Autodesk Inventor part; units mm, degrees
ref_plane "YZ Plane" through (0, 0, 0) normal (1, 0, 0) x (0, 1, 0)
ref_plane "XZ Plane" through (0, 0, 0) normal (0, 1, 0) x (-1, 0, 0)
ref_plane "XY Plane" through (0, 0, 0) normal (0, 0, 1) x (1, 0, 0)
sketch "Skizze_1" plane through (0, 0, 0) normal (0, 0, 1) x (1, 0, 0)
  arc A0 (-7.7, 0.5) -> (-7.5, 0.3) centre (-7.5, 0.5) ccw
  line L0 (-7.5, 0.3) -> (5.5, 0.3)
  arc A1 (5.5, 0.3) -> (5.7, 0.5) centre (5.5, 0.5) ccw
  line L1 (5.7, 0.5) -> (5.7, 10.1162)
  arc A2 (5.7, 10.1162) -> (5.581, 10.44) centre (5.2, 10.1162) ccw
  line L2 (5.581, 10.44) -> (4.1497, 12.1238)
  arc A3 (4.1497, 12.1238) -> (3.7688, 12.3) centre (3.7688, 11.8) ccw
  line L3 (3.7688, 12.3) -> (-7.2, 12.3)
  arc A4 (-7.2, 12.3) -> (-7.7, 11.8) centre (-7.2, 11.8) ccw
  line L4 (-7.7, 11.8) -> (-7.7, 0.5)
extrude "Extrusion1" add sketch "Skizze_1" along normal blind 7
sketch "Skizze_2" plane through (0, 0, 7) normal (0, 0, 1) x (1, 0, 0)
  line L0 (4.2, 0) -> (5.5, 0)
  arc A0 (5.5, 0) -> (5.7, 0.2) centre (5.5, 0.2) ccw
  line L1 (5.7, 0.2) -> (5.7, 0.5)
  line L2 (5.7, 0.5) -> (4.2, 0.5)
  line L3 (4.2, 0.5) -> (4.2, 0)
extrude "Extrusion2" add sketch "Skizze_2" against normal blind 0.8
pattern_linear "Rectangular Pattern1" count 2 spacing 3.5 along (0, 0, -1) of "Extrusion2"
sketch "Skizze_4" plane through (0, 0, 7) normal (0, 0, 1) x (1, 0, 0)
  line L0 (-7.7, 1) -> (-7.7, 0.2)
  arc A0 (-7.7, 0.2) -> (-7.5, 0) centre (-7.5, 0.2) ccw
  line L1 (-7.5, 0) -> (-5.7, 0)
  line L2 (-5.7, 0) -> (-5.7, 1)
  line L3 (-5.7, 1) -> (-7.7, 1)
extrude "Extrusion3" add sketch "Skizze_4" against normal blind 0.8
pattern_linear "Rectangular Pattern2" count 2 spacing 3.5 along (0, 0, -1) of "Extrusion3"
sketch "Skizze_6" plane through (0, 0, 7) normal (0, 0, 1) x (1, 0, 0)
  line L0 (-3.4, 0) -> (2.3, 0)
  line L1 (2.3, 0) -> (2.3, 1)
  line L2 (2.3, 1) -> (-3.4, 1)
  line L3 (-3.4, 1) -> (-3.4, 0)
extrude "Extrusion4" add sketch "Skizze_6" against normal blind 0.8
pattern_linear "Rectangular Pattern3" count 2 spacing 3.5 along (0, 0, -1) of "Extrusion4"
sketch "Skizze_8" plane through (0, 0, 0) normal (0, 0, 1) x (1, 0, 0)
  circle A0 centre (4.3, 1.6) radius 0.6
extrude "Extrusion5" add sketch "Skizze_8" against normal blind 1.5
sketch "Skizze_9" plane through (0, 0, 0) normal (0, 0, 1) x (1, 0, 0)
  circle A0 centre (4.3, 4.7) radius 0.6
extrude "Extrusion6" add sketch "Skizze_9" against normal blind 1.5
sketch "Skizze_10" plane through (0, 0, 0) normal (0, 0, 1) x (1, 0, 0)
  circle A0 centre (4.3, 8.3) radius 0.6
extrude "Extrusion7" add sketch "Skizze_10" against normal blind 1.5
sketch "Skizze_11" plane through (0, 0, 0) normal (0, 0, 1) x (1, 0, 0)
  circle A0 centre (-6, 1.6) radius 0.5
extrude "Extrusion8" add sketch "Skizze_11" against normal blind 1.5
sketch "Skizze_12" plane through (0, 0, 0) normal (0, 0, 1) x (1, 0, 0)
  circle A0 centre (-6, 3.4) radius 0.5
extrude "Extrusion9" add sketch "Skizze_12" against normal blind 1.5
sketch "Skizze_13" plane through (0, 0, 0) normal (0, 0, 1) x (1, 0, 0)
  circle A0 centre (-6.5, 8.9) radius 0.5
extrude "Extrusion10" add sketch "Skizze_13" against normal blind 1.5
sketch "Skizze_14" plane through (0, 0, 0) normal (0, 0, 1) x (1, 0, 0)
  circle A0 centre (-6.5, 10.8) radius 0.5
extrude "Extrusion11" add sketch "Skizze_14" against normal blind 1.5
sketch "Skizze_15" plane through (0, 0, 0) normal (0, 0, 1) x (1, 0, 0)
  arc A0 (-7.7, 0.2) -> (-7.5, 0) centre (-7.5, 0.2) ccw
  line L0 (-7.5, 0) -> (-5.7, 0)
  line L1 (-5.7, 0) -> (-5.7, 0.3)
  line L2 (-5.7, 0.3) -> (-3.4, 0.3)
  line L3 (-3.4, 0.3) -> (-3.4, 0)
  line L4 (-3.4, 0) -> (2.3, 0)
  line L5 (2.3, 0) -> (2.3, 0.3)
  line L6 (2.3, 0.3) -> (4.2, 0.3)
  line L7 (4.2, 0.3) -> (4.2, 0)
  line L8 (4.2, 0) -> (5.5, 0)
  arc A1 (5.5, 0) -> (5.7, 0.2) centre (5.5, 0.2) ccw
  line L9 (5.7, 0.2) -> (5.7, 10.1162)
  arc A2 (5.7, 10.1162) -> (5.581, 10.44) centre (5.2, 10.1162) ccw
  line L10 (5.581, 10.44) -> (4.1497, 12.1238)
  arc A3 (4.1497, 12.1238) -> (3.7688, 12.3) centre (3.7688, 11.8) ccw
  line L11 (3.7688, 12.3) -> (-7.2, 12.3)
  arc A4 (-7.2, 12.3) -> (-7.7, 11.8) centre (-7.2, 11.8) ccw
  line L12 (-7.7, 11.8) -> (-7.7, 0.2)
extrude "Extrusion12" add sketch "Skizze_15" against normal blind 1.4
sketch "Skizze_16" plane through (0, 0, 0) normal (0, 0, 1) x (1, 0, 0)
  line L0 (-5.8, 12.3) -> (-5.5, 12)
  line L1 (-5.5, 12) -> (-5.5, 10.8)
  line L2 (-5.5, 10.8) -> (-2.6, 10.8)
  line L3 (-2.6, 10.8) -> (-2.6, 12)
  line L4 (-2.6, 12) -> (-2.3, 12.3)
  line L5 (-2.3, 12.3) -> (-5.8, 12.3)
extrude "Extrusion13" cut sketch "Skizze_16" along normal blind 3.2
pattern_linear "Rectangular Pattern4" count 2 spacing 3.5 along (0, 0, 1) of "Extrusion13"
sketch "Skizze_18" plane through (0, 0, 0) normal (1, 0, 0) x (0, 1, 0)
  line L0 (10.8, 3.2) -> (10.8, 2.9)
  line L1 (10.8, 2.9) -> (12, 2.9)
  line L2 (12, 2.9) -> (12.3, 3.2)
  line L3 (12.3, 3.2) -> (10.8, 3.2)
extrude "Extrusion14" add sketch "Skizze_18" against normal blind 6
pattern_linear "Rectangular Pattern5" count 2 spacing 3.5 along (0, 0, 1) of "Extrusion14"
sketch "Skizze_20" plane through (-0.9, 0, 0) normal (1, 0, 0) x (0, 0, -1)
  line L0 (-3.2, 12.3) -> (-2.6, 10.3)
  line L1 (-2.6, 10.3) -> (-0.8, 10.3)
  line L2 (-0.8, 10.3) -> (0, 12.3)
  line L3 (0, 12.3) -> (-3.2, 12.3)
extrude "Extrusion15" cut sketch "Skizze_20" along normal blind 4.1
pattern_linear "Rectangular Pattern6" count 2 spacing 3.5 along (0, 0, 1) of "Extrusion15"
sketch "Skizze_22" plane through (0, 0, 0) normal (0, 0, 1) x (1, 0, 0)
  line L0 (-0.9, 9.8) -> (3.2, 9.8)
  line L1 (3.2, 9.8) -> (3.2, 12.3)
  line L2 (3.2, 12.3) -> (2.7, 10.3)
  line L3 (2.7, 10.3) -> (-0.35, 10.3)
  line L4 (-0.35, 10.3) -> (-0.9, 12.3)
  line L5 (-0.9, 12.3) -> (-0.9, 9.8)
extrude "Extrusion16" add sketch "Skizze_22" along normal blind 7
sketch "Skizze_23" plane through (-0.9, 0, 0) normal (1, 0, 0) x (0, 0, -1)
  line L0 (-1.7, 10.3) -> (-1.7, 12.3)
  line L1 (-1.7, 12.3) -> (-0.7, 12.3)
  line L2 (-0.7, 12.3) -> (-1, 10.3)
  line L3 (-1, 10.3) -> (-1.7, 10.3)
  line L4 (-1.7, 10.3) -> (-1.7, 12.3)
revolve "Revolution1" cut sketch "Skizze_23" angle 360 about axis through (-0.9, 10.3, 1.7) along (0, -1, 0)
pattern_linear "Rectangular Pattern7" count 2 spacing 3.5 along (0, 0, 1) of "Revolution1"
sketch "Skizze_24" plane through (-0.9, 0, 0) normal (1, 0, 0) x (0, 0, -1)
  line L0 (-2.7, 12.3) -> (-2.4, 10.3)
  line L1 (-2.4, 10.3) -> (-1, 10.3)
  line L2 (-1, 10.3) -> (-0.7, 12.3)
  line L3 (-0.7, 12.3) -> (-2.7, 12.3)
extrude "Extrusion17" cut sketch "Skizze_24" along normal blind 1
pattern_linear "Rectangular Pattern8" count 2 spacing 3.5 along (0, 0, 1) of "Extrusion17"
sketch "Skizze_27" plane through (0, 0.3, 0) normal (0, 1, 0) x (1, 0, 0)
  line L0 (-0.3, -1.35) -> (-0.3, -2.15)
  line L1 (-0.3, -2.15) -> (0.3, -2.15)
  line L2 (0.3, -2.15) -> (0.3, -1.35)
  line L3 (0.3, -1.35) -> (-0.3, -1.35)
extrude "Extrusion18" add sketch "Skizze_27" against normal blind 3.7
pattern_linear "Rectangular Pattern9" count 2 spacing 3.5 along (0, 0, 1) of "Extrusion18"
sketch "Sketch20" plane through (-0.3, -3.4, 5.65) normal (0, -1, 0) x (1, 0, 0)
  line L0 (0, 0) -> (0.6, 0) construction
  line L1 (0.6, -0.8) -> (0, -0.8) construction
  line L2 (0, -3.5) -> (0.6, -3.5) construction
  line L3 (0.6, -4.3) -> (0, -4.3) construction
  line L4 (0, -3.5) -> (0.6, -4.3) construction
  line L5 (0, 0) -> (0.6, -0.8) construction
  circle A0 centre (0.3, -0.4) radius 0.25
  circle A1 centre (0.3, -3.9) radius 0.25
  point P0 (0.3, -5.65)
  dimension "d91" = 0.5
extrude "Extrusion19" cut sketch "Sketch20" against normal blind 0.5
properties part number "739-302"
CAD build for the part. Positions are in the model's coordinates, mm. A direction names the side the tool comes from. Coordinates: 2 decimals unless noted, no trailing zeros. Write each loop counter-clockwise with the first axis right and the second up, starting at its lowest first coordinate (ties: lowest second). Pieces come first, ordered by that corner, then holes.
(1) Flat gauge pins, fed straight in: pin 1 (8 mm diameter, centred on x = 4.5, y = 9.5, fed in from -Z); pin 2 (1.5 mm diameter, centred on x = -6.5, z = -1, fed in from -Y); pin 3 (1 mm diameter, centred on y = -0.5, z = 5.5, fed in from -X); pin 4 (2 mm diameter, centred on x = 3, z = 5, fed in from -Y). Where does each tip first touch, or does it go through?
(2) Cut at C-C, the plane x = -4.75. List the corners of the cut face in (y, z).
(3) Cut at B-B, the plane x = 3. List the corners of the cut face in (y, z), and give its area (3 significant figures).
(4) 3-axis set-ups, long thin cutter, end or side, ignore diameter. For faces 1 (the face through (5.7, 5, 3)), 2 (the face through (1.1, 11.3, 2.9)): which of +Z, -Z, +X, -X, +Y, -Y reach the whole face in a straight line?
(5) Cut at A-A, the plane y = -2. List the corners of the cut face in (x, z), and give its area (3 significant figures).
(6) Drill centre lines: probe 1 along Z at (x, y) = (0, -3.05); probe 2 along Y at (x, z) = (-0.25, -0.75); probe 3 along Z at (x, y) = (-1.5, 11.75). Where is each one in solid material? Low to high.
Geometry says:
1. pin 1: stops at z = -1.5
1. pin 2: stops at y = 0
1. pin 3: stops at x = -0.3
1. pin 4: stops at y = 0.3
2. outline: (0.3, -1.4) - (12.3, -1.4) - (12.3, 0) - (10.8, 0) - (10.8, 2.9) - (12, 2.9) - (12.3, 3.2) - (12.3, 3.5) - (10.8, 3.5) - (10.8, 6.4) - (12, 6.4) - (12.3, 6.7) - (12.3, 7) - (0.3, 7) - close
3. outline: (0.3, -1.4) - (12.3, -1.4) - (12.3, 0) - (11.5, 0.32) - (11.5, 2.96) - (12.3, 3.2) - (12.3, 3.5) - (11.5, 3.82) - (11.5, 6.46) - (12.3, 6.7) - (12.3, 7) - (0.3, 7) - close
3. area: 96.1 mm2
4. face 1: +Z, -Z, +X, +Y, -Y
4. face 2: +Y
5. outline: (-0.3, 1.35) - (0.3, 1.35) - (0.3, 2.15) - (-0.3, 2.15) - close; (-0.3, 4.85) - (0.3, 4.85) - (0.3, 5.65) - (-0.3, 5.65) - close
5. area: 0.960 mm2
6. probe 1: z = 1.35 to 1.5, 2 to 2.15, 4.85 to 5, 5.5 to 5.65
6. probe 2: y = 0 to 12.3
6. probe 3: z = -1.4 to 1.01, 2.39 to 4.51, 5.89 to 7
